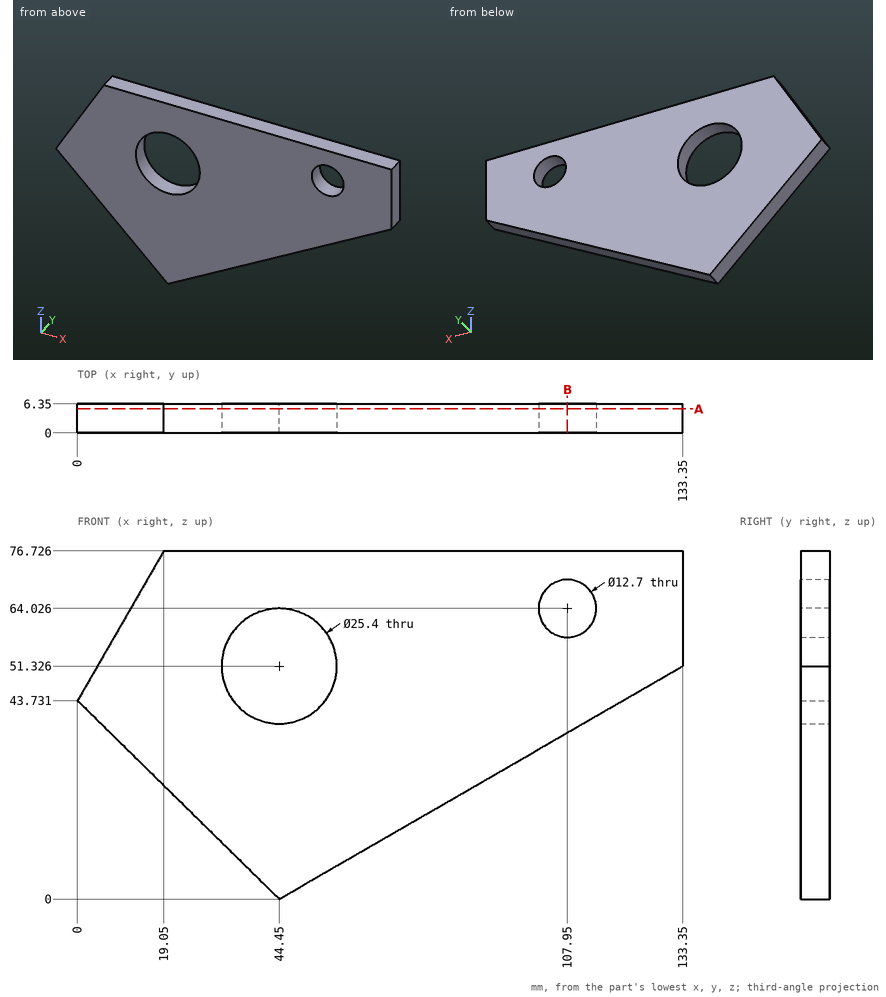
Check sheet for the drawn part. Datum: minimum x, y, z corner. Units: mm. Coordinates: 2 decimals unless noted, no trailing zeros. Order: outer loops, then holes, each group sorted by start corner. A loop starts at its lowest first (then second) coordinate and runs counter-clockwise, first axis right, second up. Notation, with made-up numbers: M 76.5,8 L 93.5,8 A9 ccw 93.5,24 Z; hole C -16.75,-8 d2. An arc over 180 degrees is marked long. One line per question, with ' | ' between items. Start each with the question number.
Item 1: Gauge pin test, flat end, axial feed: pin 1 (1 mm diameter, centred on x = 119, z = 60.5, fed in from -Y). Record the tip position at first contact, or that the pin passes through.
Item 2: Cross-section at A-A on y = 5.25. Enter the section's corners in (x, z), then the cut area to 3 significant figures.
Item 3: Material ranges on L1, parallel to X at y = 3, z = 48 (1 decimal); L2, parallel to Z at x = 111.5, y = 1.5 (1 decimal); L3, parallel to X at y = 2.5, z = 51 (1 decimal), recorded low to high. Write a range as [from, to].
Item 4: Cross-section at B-B on x = 107.95. Enter the section's corners in (y, z), then the cut area to 3 significant figures.
Findings:
1) pin 1: stops at y = 0
2) outline: M 0,43.73 L 44.45,0 L 133.35,51.33 L 133.35,76.73 L 19.05,76.73 Z; hole C 44.45,51.33 d25.4; hole C 107.95,64.03 d12.7 | area: 6,030 mm²
3) L1: x = [2.5, 32.2], [56.7, 127.6] | L2: z = [38.7, 58.8], [69.3, 76.7] | L3: x = [4.2, 31.8], [57.1, 132.8]
4) outline: M 0,36.66 L 6.35,36.66 L 6.35,57.68 L 0,57.68 Z; M 0,70.38 L 6.35,70.38 L 6.35,76.73 L 0,76.73 Z | area: 174 mm²
